Geometry: see drawing. Coordinates: mm, zero at the bounding-box minimum. A direction names the side the tool comes from. Round coordinates to 2 decimals unless told otherwise and drop trailing zeros. Order: outer loops, then holes, each group sorted by start corner. A loop starts at its lowest first (then second) coordinate and runs counter-clockwise, first axis right, second up. Notation, with made-up numbers: (80, -18.5) -> (118, -18.5) arc R22 ccw to (118, 3.5) -> close; hole circle Ø7 at (43, 28.5). An arc over 180 degrees is marked (long way). Use a Markdown table: item, result.
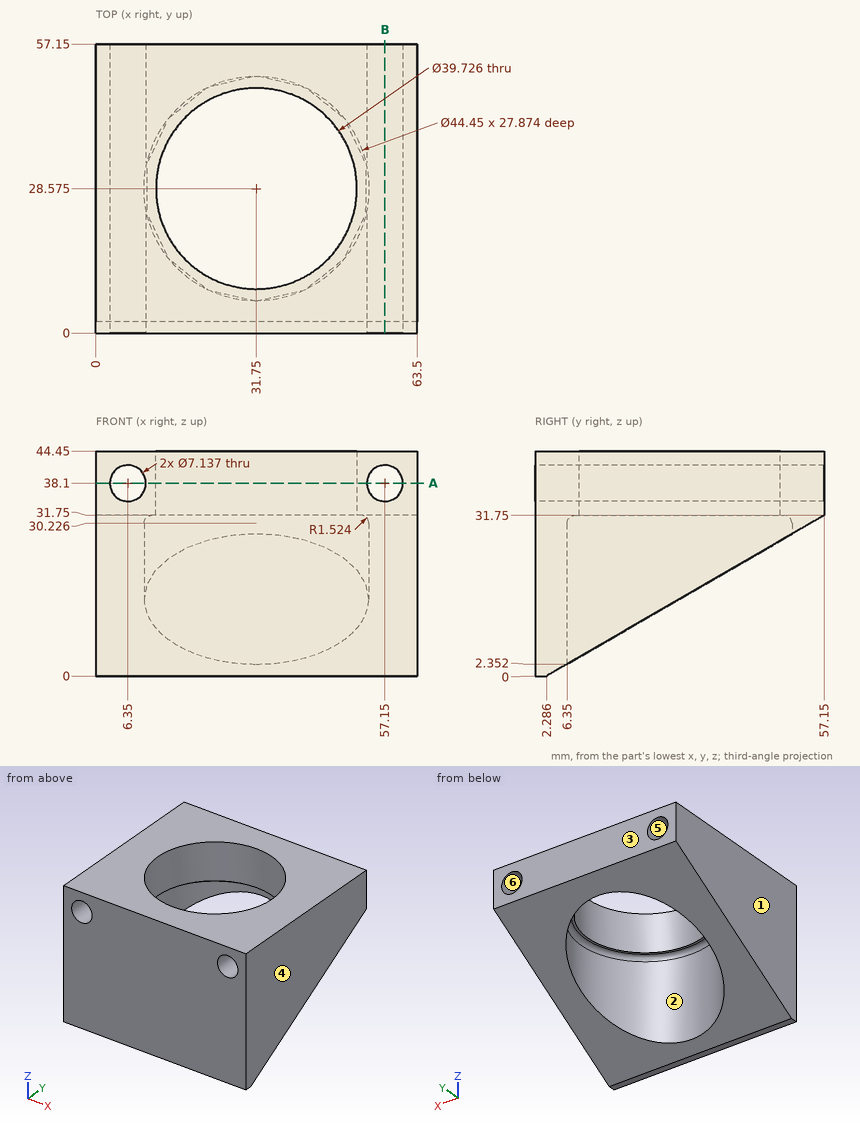
1) Cut plane B-B on x = 57.15. Return loops of the section in (y, z), and give its area (3 significant figures).
Answer key:
| item | result |
|---|---|
| outline | (0, 0) -> (2.29, 0) -> (57.15, 31.75) -> (57.15, 34.53) -> (0, 34.53) -> close; (0, 41.67) -> (57.15, 41.67) -> (57.15, 44.45) -> (0, 44.45) -> close |
| area | 1,260 mm^2 |
2) Draft query along X for the marked faces 3, 4, 5 and 6. Return one class per face: released by +X, released by -X, zero draft, split by the parting line, or undercut.
Answer key:
| item | result |
|---|---|
| face 3 | zero draft |
| face 4 | released by +X |
| face 5 | undercut |
| face 6 | undercut |
3) Contact query for flat-ended pins moving along their axis: P1, Ø2, axis at x = 10, z = 9, coming from the -Y side; P2, Ø6.5, axis at x = 57.15, z = 38.1, coming from the +Y side; P3, Ø1.5, axis at x = 54.5, y = 26, coming from the -Z side. Output: stop coordinate, or through.
Answer key:
| item | result |
|---|---|
| P1 | stops at y = 0 |
| P2 | passes through |
| P3 | stops at z = 13.29 |
4) Set-up query: the marked faces 1 and 2. Return all of +Z, -Z, +X, -X, +Y, -Y with unobstructed straight access to the full face (end or side cutting, diameter ignored); none if empty.
Answer key:
| item | result |
|---|---|
| face 1 | +Z, -Z, -X, +Y, -Y |
| face 2 | -Z |
5) Cut plane A-A on z = 38.1. State how many separate pieces and enclosed holes the cut face has, and give its area (3 significant figures).
Answer key:
| item | result |
|---|---|
| separate pieces | 3 |
| enclosed holes | 1 |
| area | 1,570 mm^2 |
6) Ray query, probe 1 along Y at (x, z) = (32, 42); probe 2 along X at (y, z) = (28.5, 21) (1 decimal); probe 3 along X at (y, z) = (29, 38.5). Return the intervals inside material, ascending.
Answer key:
| item | result |
|---|---|
| probe 1 | y = 0 to 8.71, 48.44 to 57.15 |
| probe 2 | x = 0 to 9.5, 54 to 63.5 |
| probe 3 | x = 0 to 2.8, 9.9 to 11.89, 51.61 to 53.6, 60.7 to 63.5 |
